Can you work these out from the model? Positions are in its coordinate system, mm. Give positions to 0.01 mm unless a question says otherwise; leave off trailing zeros. Order: outer loops, then holes, each group sorted by start corner. A loop starts at its lowest first (then second) coordinate and runs counter-clockwise, first axis right, second up. Notation, with made-up numbers: M -31.75,15 L -17.75,15 A34 cw -17.75,48 Z; hole C 14.5,-14.5 d7. An arc over 180 degrees is marked long. Use one line per item in the form item = value. Start each with the question number.
1. I want a section at C-C, the plane y = 249.5. List the corners of the cut face in (x, z) for me.
2. I want a section at A-A, the plane x = 3.9. List the corners of the cut face in (y, z) for me, and give its area (3 significant figures).
3. I need wall thicknesses on L1, parallel to Y at x = 4.95, z = 231; L2, parallel to Y at x = 3.8, z = 413.5. Which ranges of each line are inside material? Lowest first, please.
4. I want a section at B-B, the plane z = 427. List the corners of the cut face in (x, y) for me.
5. Will these pins go through, and if not, where does the flat tip stop? P1, Ø6.5, axis at y = 239.15, z = 213.77, coming from the -X side; P2, Ø2, axis at x = 2.5, y = 213, coming from the +Z side.
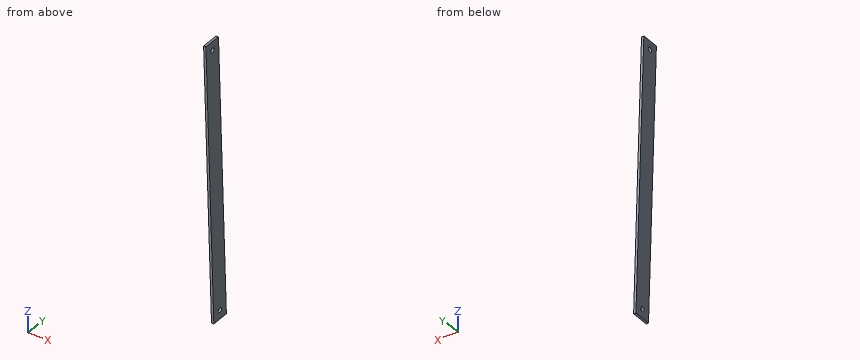
```python
from build123d import *

# Parameters (mm, degrees)
SKETCH1_R           = 4
BOSS_EXTRUDE1_DEPTH = 4


with BuildPart() as part:
    # Sketch1 → Boss-Extrude1 (new body)
    with BuildSketch(Plane(origin=(1.4, 0, 0), x_dir=(0, -1, 0), z_dir=(-1, 0, 0))):
        with BuildLine():
            Line((-254.739115199, 199.375774934), (-224.762842625, 198.182844675))
            Line((-224.762842625, 198.182844675), (-205.908265943, 671.965721187))
            ThreePointArc((-205.908265943, 671.965721187), (-206.131039779, 672.570516328), (-206.716219414, 672.840646182))
            Line((-206.716219414, 672.840646182), (-235.009613521, 673.966604918))
            ThreePointArc((-235.009613521, 673.966604918), (-235.614408661, 673.743831082), (-235.884538516, 673.158651447))
            Line((-235.884538516, 673.158651447), (-254.739115199, 199.375774934))
        make_face()
        with Locations(Location((-221.459381597, 658.415489264, 0), (0, 0, 270))):
            Circle(SKETCH1_R, mode=Mode.SUBTRACT)
        with Locations(Location((-239.154513782, 213.767446091, 0), (0, 0, 270))):
            Circle(SKETCH1_R, mode=Mode.SUBTRACT)
    extrude(amount=-BOSS_EXTRUDE1_DEPTH)


solid = part.part
```
Check result:
q1.outline = M 1.4,199.17 L 5.4,199.17 L 5.4,331.03 L 1.4,331.03 Z
q2.outline = M 205.91,671.97 L 224.76,198.18 L 254.74,199.38 L 235.88,673.16 A0.84 ccw 235.01,673.97 L 206.72,672.84 A0.84 ccw Z; hole C 221.46,658.42 d8; hole C 239.15,213.77 d8
q2.area = 14,100 mm2
q3.L1 = 223.46 to 253.48
q3.L2 = 216.19 to 246.22
q4.outline = M 1.4,215.66 L 5.4,215.66 L 5.4,245.68 L 1.4,245.68 Z
q5.P1 = through
q5.P2 = 673.13
